Verification items for the finished model (mm, model axes). A direction names the side the tool comes from. Round coordinates to 2 decimals unless told otherwise and drop trailing zeros. Order: outer loops, then holes, each group sorted by start corner. A loop starts at its lowest first (then second) coordinate and runs counter-clockwise, first axis right, second up. Notation, with made-up numbers: (23.25, -6) -> (63.25, -6) arc R22 cw to (63.25, 3) -> close; hole circle Ø3 at (25, -15.75). An arc over 180 degrees is marked (long way). Put each result on its own line as item: value.
from build123d import *

# Parameters (mm, degrees)
SKETCH_1_W          = 45
SKETCH_1_H          = 20
EXTRUDE_1_DEPTH     = 1.2
SKETCH_2_R          = 8
EXTRUDE_2_DEPTH     = 15
EXTRUDE_3_DEPTH     = 5
CUT_EXTRUDE_START   = 15
SKETCH_5_R          = 7
CUT_EXTRUDE_1_DEPTH = 1


with BuildPart() as part:
    # 草图1 → 凸台-拉伸1 (new body)
    with BuildSketch(Plane.XY):
        Rectangle(SKETCH_1_W, SKETCH_1_H)
    extrude(amount=EXTRUDE_1_DEPTH)

    # 草图2 → 凸台-拉伸2 (add)
    with BuildSketch(Plane.XY):
        with Locations(Location((-13.5, 0, 0), (0, 0, 180))):
            Circle(SKETCH_2_R)
        with Locations(Location((13.5, 0, 0), (0, 0, 180))):
            Circle(SKETCH_2_R)
    extrude(amount=EXTRUDE_2_DEPTH)

    # 草图3 → 凸台-拉伸3 (add)
    with BuildSketch(Plane.XY):
        with BuildLine():
            Line((-3, 9), (3, 9))
            ThreePointArc((3, 9), (4.5, 7.5), (3, 6))
            Line((3, 6), (-3, 6))
            ThreePointArc((-3, 6), (-4.5, 7.5), (-3, 9))
        make_face()
    extrude(amount=EXTRUDE_3_DEPTH)

    # 草图5 → 切除-拉伸1 (cut)
    with BuildSketch(Plane.XY.offset(CUT_EXTRUDE_START)):
        with Locations((-13.5, 0)):
            Circle(SKETCH_5_R)
        with Locations((13.5, 0)):
            Circle(SKETCH_5_R)
    extrude(amount=-CUT_EXTRUDE_1_DEPTH, mode=Mode.SUBTRACT)


solid = part.part
Item 1: Section check B-B on y = 0. Record the boundary of the cut face in (x, z), then the cut area to 3 significant figures.
Check sheet entries:
outline: (-22.5, 0) -> (22.5, 0) -> (22.5, 1.2) -> (21.5, 1.2) -> (21.5, 15) -> (20.5, 15) -> (20.5, 14) -> (6.5, 14) -> (6.5, 15) -> (5.5, 15) -> (5.5, 1.2) -> (-5.5, 1.2) -> (-5.5, 15) -> (-6.5, 15) -> (-6.5, 14) -> (-20.5, 14) -> (-20.5, 15) -> (-21.5, 15) -> (-21.5, 1.2) -> (-22.5, 1.2) -> close
area: 468 mm^2
Item 2: Release check for a two-part mould opening along X. For faces 5 (the flat face through (22.5, 0, 1)), 6 (the flat face through (0, -10, 1)), 7 (the cylindrical face through (6.507, 0.308, 14.507)) record: +X half, -X half, draft (parallel to the pull), parting line (faces both ways), or undercut.
Check sheet entries:
face 5: +X half
face 6: draft
face 7: undercut
Item 3: Tool access check on faces 1 (the flat face through (0, 9, 3)), 2 (the flat face through (0, 8, 5)), 3 (the cylindrical face through (4.5, 7.5, 3.1)), 4 (the flat face through (0, 6, 3)). Record the directions out of +Z, -Z, +X, -X, +Y, -Y that give a thin tool (end or side, any length) a straight path to the whole face; none if there is none.
Check sheet entries:
face 1: +Z, +X, -X, +Y
face 2: +Z, +Y, -Y
face 3: +Z
face 4: +Z, -Y
Item 4: Section check A-A on x = -13.5. Record the boundary of the cut face in (y, z), then the cut area to 3 significant figures.
Check sheet entries:
outline: (-10, 0) -> (10, 0) -> (10, 1.2) -> (8, 1.2) -> (8, 15) -> (7, 15) -> (7, 14) -> (-7, 14) -> (-7, 15) -> (-8, 15) -> (-8, 1.2) -> (-10, 1.2) -> close
area: 231 mm^2
Item 5: Material ranges on L1, parallel to Y at x = 13.5, z = 14.75; L2, parallel to Z at x = -19.5, y = 8; L3, parallel to Z at x = 15, y = -4.25, recorded low to high. Write a range as [from, to].
Check sheet entries:
L1: y = [-8, -7], [7, 8]
L2: z = [0, 1.2]
L3: z = [0, 14]
Item 6: Gauge pin test, flat ends, axial feed: pin 1 Ø1 at (x, z) = (4, 3) entering from -Y; pin 2 Ø2 at (y, z) = (-1, 7.5) entering from -X; pin 3 Ø1.1 at (x, z) = (0, 3) entering from -Y. Record the tip position at first contact, or that the pin passes through.
Check sheet entries:
pin 1: stops at y = 6.09
pin 2: stops at x = -21.5
pin 3: stops at y = 6
Item 7: Section check D-D on y = 7.5. Record the boundary of the cut face in (x, z).
Check sheet entries:
outline: (-22.5, 0) -> (22.5, 0) -> (22.5, 1.2) -> (16.28, 1.2) -> (16.28, 15) -> (10.72, 15) -> (10.72, 1.2) -> (4.5, 1.2) -> (4.5, 5) -> (-4.5, 5) -> (-4.5, 1.2) -> (-10.72, 1.2) -> (-10.72, 15) -> (-16.28, 15) -> (-16.28, 1.2) -> (-22.5, 1.2) -> close
Item 8: Section check C-C on z = 6.5. Record the boundary of the cut face in (x, y).
Check sheet entries:
outline: circle Ø16 at (-13.5, 0); circle Ø16 at (13.5, 0)
